Source: CAD feature listing. Evaluate the final solid. Frame: model axes, mm. Face numbers are marked on the shaded views. A direction names the side the tool comes from. Coordinates: 2 decimals unless noted, no trailing zeros. Order: outer loops, then holes, each group sorted by start corner. A loop starts at its lowest first (then second) coordinate and runs counter-clockwise, first axis right, second up.
Item 1: Contact query for flat-ended pins moving along their axis: P1, Ø11.5, axis at x = -135.52, z = -25, coming from the -Y side; P2, Ø14.5, axis at x = 132.5, y = -105.5, coming from the -Z side; P3, Ø4, axis at y = -40.5, z = 8.5, coming from the -X side; P4, Ø1, axis at x = -24.5, y = -92, coming from the +Z side. Output: stop coordinate, or through.
Item 2: Section D-D on y = -25.5. Return the cut outline in (x, z).
Item 3: Section A-A on x = 0. Return the cut outline in (y, z).
Item 4: Reachability of the marked faces 4 and 5 from +Z, -Z, +X, -X, +Y, -Y: full face, straight path, thin tool, end or side. Return the list, or none.
Item 5: Ray query, line 1 (X direction, y = -67, z = 0); line 2 (X direction, y = -156, z = -25); line 3 (Z direction, x = 135, y = -80). Return the intervals inside material, ascending.
Item 6: Mould query, pull axis X, two halves, no side actions, for the marked faces 1, 2 and 3. Classes: released by +X, released by -X, zero draft, split by the parting line, or undercut.
Item 7: Section C-C on z = -25. State how many separate pieces and enclosed holes the cut face has, then the cut area to 3 significant figures.
Item 8: Section B-B on y = -127.5. Return the cut outline in (x, z).
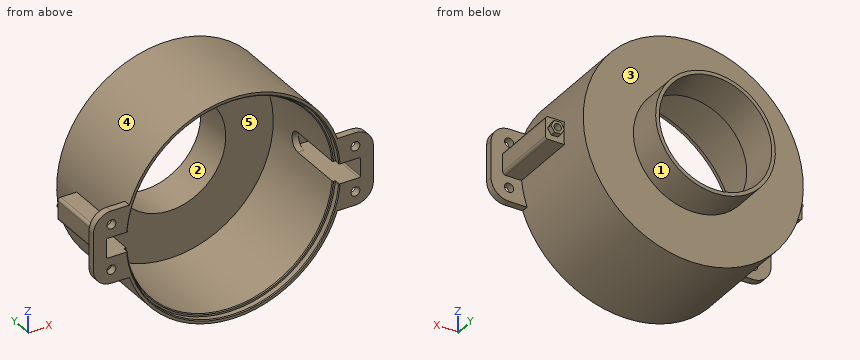
from build123d import *

# Parameters (mm, degrees)
CHAMFER1_SIZE           = 1
CUT_EXTRUDE1_DEPTH      = 236.563420335
CUT_EXTRUDE1_DEPTH_BACK = 236.563420335
BOSS_EXTRUDE2_START     = -160
BOSS_EXTRUDE2_DEPTH     = 85
BOSS_EXTRUDE3_START     = -3
BOSS_EXTRUDE3_DEPTH     = 3
FILLET1_R               = 1.5
FILLET2_R               = 3
FILLET1_OF_MIRROR1_R    = 1.5
FILLET2_OF_MIRROR1_R    = 3
SKETCH6_R               = 5
BOSS_EXTRUDE4_DEPTH     = 8
FILLET3_R               = 20
SKETCH7_R               = 4
CUT_EXTRUDE2_DEPTH      = 10
BOSS_EXTRUDE5_START     = 6
SKETCH8_R               = 4
BOSS_EXTRUDE5_DEPTH     = 6


with BuildPart() as part:
    # Sketch1 → Revolve1 (revolve)
    with BuildSketch(Plane.XY, mode=Mode.PRIVATE) as revolve1_sk:
        Polygon((-122.25, -160), (-118.25, -160), (-118.25, -153), (-115.25, -153), (-115.25, -45), (-62.5, -45), (-62.5, 0), (-66.5, 0), (-66.5, -40), (-122.25, -40), align=None)
    revolve(revolve1_sk.sketch.rotate(Axis((0, -155, 0), (0, 1, 0)), 270), axis=Axis((0, -155, 0), (0, 1, 0)))

    # Chamfer1
    chamfer1_edges = [part.edges().sort_by_distance(p)[0] for p in [
        (0, -153, 115.25),
        (0, -160, 118.25),
    ]]
    chamfer(chamfer1_edges, length=CHAMFER1_SIZE)

    # Sketch3 → Cut-Extrude1 (cut, two sides: drawn at the far end of the back side and taken through both)
    with BuildSketch(Plane(origin=(0, 0, 0), x_dir=(0, 0, -1), z_dir=(1, 0, 0)).offset(-CUT_EXTRUDE1_DEPTH_BACK)):
        with BuildLine():
            Line((-11, -160), (-11, -90))
            ThreePointArc((-11, -90), (0, -79), (11, -90))
            Line((11, -90), (11, -160))
            ThreePointArc((11, -160), (0, -171), (-11, -160))
        make_face()
    extrude(amount=CUT_EXTRUDE1_DEPTH + CUT_EXTRUDE1_DEPTH_BACK, mode=Mode.SUBTRACT)

    # Sketch2 → Boss-Extrude2 (add)
    with BuildSketch(Plane(origin=(34.652885487, 0, -427.94626462), x_dir=(1, 0, 0), z_dir=(0, 1, 0)).offset(BOSS_EXTRUDE2_START)):
        Polygon((107.934581958, -415.44626462), (82.934581958, -415.44626462), (82.934581958, -416.94626462), (106.434581958, -416.94626462), (106.434581958, -438.94626462), (82.934581958, -438.94626462), (82.934581958, -440.44626462), (107.934581958, -440.44626462), align=None)
    boss_extrude2 = extrude(amount=BOSS_EXTRUDE2_DEPTH)

    # Sketch5 → Boss-Extrude3 (add)
    with BuildSketch(Plane(origin=(0, -75, 0), x_dir=(1, 0, 0), z_dir=(0, 1, 0)).offset(BOSS_EXTRUDE3_START)):
        with BuildLine():
            Line((141.087467444, -11), (141.087467444, 11))
            Line((141.087467444, 11), (121.754106707, 11))
            ThreePointArc((121.754106707, 11), (122.125963752, 5.505586031), (122.25, 0))
            ThreePointArc((122.25, 0), (122.125963752, -5.505586031), (121.754106707, -11))
            Line((121.754106707, -11), (141.087467444, -11))
        make_face()
    boss_extrude3 = extrude(amount=BOSS_EXTRUDE3_DEPTH)

    # Fillet1
    fillet1_edges = [part.edges().sort_by_distance(p)[0] for p in [
        (141.087467444, -119, 11),
        (141.087467444, -119, -11),
    ]]
    fillet(fillet1_edges, radius=FILLET1_R)

    # Fillet2
    fillet2_edges = [part.edges().sort_by_distance(p)[0] for p in [
        (142.587467444, -117.5, 12.5),
        (142.587467444, -117.5, -12.5),
    ]]
    fillet(fillet2_edges, radius=FILLET2_R)

    # Mirror1: Boss-Extrude2, Boss-Extrude3 across plane
    add(boss_extrude2.mirror(Plane(origin=(0, 0, 0), x_dir=(0, 0, 1), z_dir=(1, 0, 0))))
    add(boss_extrude3.mirror(Plane(origin=(0, 0, 0), x_dir=(0, 0, 1), z_dir=(1, 0, 0))))

    # Fillet1 of Mirror1
    fillet1_of_mirror1_edges = [part.edges().sort_by_distance(p)[0] for p in [
        (-141.087467444, -119, 11),
        (-141.087467444, -119, -11),
    ]]
    fillet(fillet1_of_mirror1_edges, radius=FILLET1_OF_MIRROR1_R)

    # Fillet2 of Mirror1
    fillet2_of_mirror1_edges = [part.edges().sort_by_distance(p)[0] for p in [
        (-142.587467444, -117.5, 12.5),
        (-142.587467444, -117.5, -12.5),
    ]]
    fillet(fillet2_of_mirror1_edges, radius=FILLET2_OF_MIRROR1_R)

    # Sketch6 → Boss-Extrude4 (add)
    # profile 1 of 2: a face of its own
    with BuildSketch(Plane.XZ.offset(160)):
        with BuildLine():
            Line((-155.520831455, 40), (-155.520831455, -40))
            Line((-155.520831455, -40), (-115.520831455, -40))
            ThreePointArc((-115.520831455, -40), (-119.359678094, -26.425929413), (-121.609261572, -12.5))
            Line((-121.609261572, -12.5), (-139.587467444, -12.5))
            ThreePointArc((-139.587467444, -12.5), (-141.708787788, -11.621320344), (-142.587467444, -9.5))
            Line((-142.587467444, -9.5), (-142.587467444, 9.5))
            ThreePointArc((-142.587467444, 9.5), (-141.708787788, 11.621320344), (-139.587467444, 12.5))
            Line((-139.587467444, 12.5), (-121.609261572, 12.5))
            ThreePointArc((-121.609261572, 12.5), (-119.359678094, 26.425929413), (-115.520831455, 40))
            Line((-115.520831455, 40), (-155.520831455, 40))
        make_face()
        with Locations(Location((-135.520831455, -25, 0), (0, 0, 270))):
            Circle(SKETCH6_R, mode=Mode.SUBTRACT)
        with Locations(Location((-135.520831455, 25, 0), (0, 0, 270))):
            Circle(SKETCH6_R, mode=Mode.SUBTRACT)
    # profile 2 of 2: a face of its own
    with BuildSketch(Plane.XZ.offset(160)):
        with BuildLine():
            ThreePointArc((121.609261572, -12.5), (119.359678094, -26.425929413), (115.520831455, -40))
            Line((115.520831455, -40), (155.520831455, -40))
            Line((155.520831455, -40), (155.520831455, 40))
            Line((155.520831455, 40), (115.520831455, 40))
            ThreePointArc((115.520831455, 40), (119.359678094, 26.425929413), (121.609261572, 12.5))
            Line((121.609261572, 12.5), (139.587467444, 12.5))
            ThreePointArc((139.587467444, 12.5), (141.708787788, 11.621320344), (142.587467444, 9.5))
            Line((142.587467444, 9.5), (142.587467444, -9.5))
            ThreePointArc((142.587467444, -9.5), (141.708787788, -11.621320344), (139.587467444, -12.5))
            Line((139.587467444, -12.5), (121.609261572, -12.5))
        make_face()
        with Locations(Location((135.520831455, -25, 0), (0, 0, 270))):
            Circle(SKETCH6_R, mode=Mode.SUBTRACT)
        with Locations(Location((135.520831455, 25, 0), (0, 0, 270))):
            Circle(SKETCH6_R, mode=Mode.SUBTRACT)
    extrude(amount=-BOSS_EXTRUDE4_DEPTH)

    # Fillet3
    fillet3_edges = [part.edges().sort_by_distance(p)[0] for p in [
        (-155.520831455, -156, 40),
        (-155.520831455, -156, -40),
        (155.520831455, -156, -40),
        (155.520831455, -156, 40),
    ]]
    fillet(fillet3_edges, radius=FILLET3_R)

    # Sketch7 → Cut-Extrude2 (cut)
    with BuildSketch(Plane(origin=(0, -75, 0), x_dir=(1, 0, 0), z_dir=(0, 1, 0))):
        with Locations(Location((-132.699855766, 0, 0), (0, 0, 270))):
            Circle(SKETCH7_R)
    cut_extrude2 = extrude(amount=-CUT_EXTRUDE2_DEPTH, mode=Mode.SUBTRACT)

    # Sketch8 → Boss-Extrude5 (add)
    with BuildSketch(Plane(origin=(0, -75, 0), x_dir=(1, 0, 0), z_dir=(0, 1, 0)).offset(BOSS_EXTRUDE5_START)):
        Polygon((-128.770701066, 6.394925854), (-136.273446661, 6.600210713), (-140.202601361, 0.205284859), (-136.629010467, -6.394925854), (-129.126264872, -6.600210713), (-125.197110172, -0.205284859), align=None)
        with Locations(Location((-132.699855766, 0, 0), (0, 0, 270))):
            Circle(SKETCH8_R, mode=Mode.SUBTRACT)
    boss_extrude5 = extrude(amount=-BOSS_EXTRUDE5_DEPTH)

    # Mirror2: Cut-Extrude2, Boss-Extrude5 across plane
    add(cut_extrude2.mirror(Plane(origin=(0, 0, 0), x_dir=(0, 0, 1), z_dir=(1, 0, 0))), mode=Mode.SUBTRACT)
    add(boss_extrude5.mirror(Plane(origin=(0, 0, 0), x_dir=(0, 0, 1), z_dir=(1, 0, 0))))


solid = part.part
Answer list:
1. P1: stops at y = -160
1. P2: stops at z = -12.5
1. P3: stops at x = -122.08
1. P4: stops at z = 119.87
2. outline: circle Ø133 at (0, 0); hole circle Ø125 at (0, 0)
3. outline: (-160, -122.25) - (-40, -122.25) - (-40, -66.5) - (0, -66.5) - (0, -62.5) - (-45, -62.5) - (-45, -115.25) - (-152, -115.25) - (-153, -116.25) - (-153, -118.25) - (-159, -118.25) - (-160, -119.25) - close; (-160, 119.25) - (-159, 118.25) - (-153, 118.25) - (-153, 116.25) - (-152, 115.25) - (-45, 115.25) - (-45, 62.5) - (0, 62.5) - (0, 66.5) - (-40, 66.5) - (-40, 122.25) - (-160, 122.25) - close
4. face 4: +Y
4. face 5: -Y
5. line 1: x = -122.25 to -115.25, 115.25 to 122.25
5. line 2: x = -154.89 to -140.52, -130.52 to -115.58, 115.58 to 130.52, 140.52 to 154.89
5. line 3: z = -12.5 to -11, 11 to 12.5
6. face 1: split by the parting line
6. face 2: undercut
6. face 3: zero draft
7. separate pieces: 4
7. enclosed holes: 0
7. area: 2,980 mm2
8. outline: (-142.59, -9.5) arc R3 ccw to (-139.59, -12.5) - (-121.61, -12.5) arc R122.25 ccw to (121.61, -12.5) - (139.59, -12.5) arc R3 ccw to (142.59, -9.5) - (142.59, 9.5) arc R3 ccw to (139.59, 12.5) - (121.61, 12.5) arc R122.25 ccw to (-121.61, 12.5) - (-139.59, 12.5) arc R3 ccw to (-142.59, 9.5) - close; hole (-141.09, -9.5) arc R1.5 ccw to (-139.59, -11) - (-114.72, -11) arc R115.25 ccw to (114.72, -11) - (139.59, -11) arc R1.5 ccw to (141.09, -9.5) - (141.09, 9.5) arc R1.5 ccw to (139.59, 11) - (114.72, 11) arc R115.25 ccw to (-114.72, 11) - (-139.59, 11) arc R1.5 ccw to (-141.09, 9.5) - close
